Check sheet for the modelled part. Datum: model origin and axes. Units: mm. Face numbers are marked on the shaded views. Coordinates: 2 decimals unless noted, no trailing zeros. Order: outer loops, then holes, each group sorted by start corner. A loop starts at its lowest first (then second) coordinate and runs counter-clockwise, first axis right, second up.
1. Cross-section at A-A (z = 0). Count the separate pieces of the cut face and the enclosed holes in it, then the cut area to 3 significant figures.
2. Thickness scan on line 1 (Z direction, x = -1, y = -2.75); line 2 (Y direction, x = 33, z = 2); line 3 (Z direction, x = 76.2, y = 5). Record the ranges inside material, lowest first.
3. Cross-section at B-B (x = 76.2). Enter the section's corners in (y, z).
4. Draft check along Z on the marked faces 1 and 2. Enter one of: released by +Z, released by -Z, zero draft, split by the parting line, or undercut.
5. Cross-section at D-D (z = 7.5). Enter the section's corners in (x, y), then the cut area to 3 significant figures.
6. Gauge pin test, flat ends, axial feed: pin 1 Ø7.5 at (x, z) = (25.4, 0) entering from -Y; pin 2 Ø6.5 at (x, z) = (76.2, 23.81) entering from +Y; pin 3 Ø21 at (x, z) = (-3, 0.5) entering from +Y; pin 4 Ø2 at (x, z) = (-47, 25) entering from -Y. Record the tip position at first contact, or that the pin passes through.
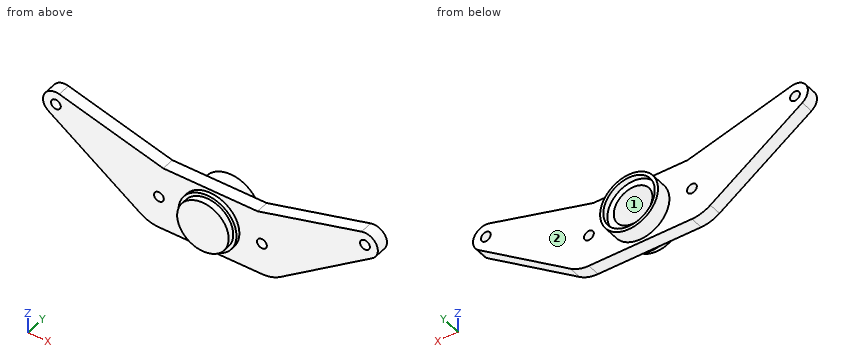
```python
from build123d import *

# Parameters (mm, degrees)
BOSS_EXTRUDE1_DEPTH    = 6.35
BOSS_EXTRUDE2_START    = -14.224
SKETCH2_R              = 14.2875
BOSS_EXTRUDE2_DEPTH    = 19.431
HOLE1_D                = 19.05
HOLE1_DEPTH            = 19.05
HOLE1_CBORE_D          = 25.4
HOLE1_CBORE_DEPTH      = 2.794
F_10_32_TAPPED_HOLE1_D = 4.826
SKETCH7_R              = 14.2875
SKETCH7_R_2            = 12.7
CUT_EXTRUDE1_DEPTH     = 3.175


with BuildPart() as part:
    # Sketch1 → Boss-Extrude1 (new body)
    with BuildSketch(Plane(origin=(0, 0, 0), x_dir=(1, 0, 0), z_dir=(0, 1, 0))):
        with BuildLine():
            Line((79.832170731, -18.603869107), (34.480426828, 13.021577233))
            ThreePointArc((34.480426828, 13.021577233), (30.159101093, 15.14485331), (25.4, 15.875))
            Line((25.4, 15.875), (-25.4, 15.875))
            ThreePointArc((-25.4, 15.875), (-30.159101093, 15.14485331), (-34.480426828, 13.021577233))
            Line((-34.480426828, 13.021577233), (-79.832170731, -18.603869107))
            ThreePointArc((-79.832170731, -18.603869107), (-81.949664243, -26.507655114), (-74.520111094, -29.936262999))
            Line((-74.520111094, -29.936262999), (-23.262053626, -15.875))
            Line((-23.262053626, -15.875), (23.262053626, -15.875))
            Line((23.262053626, -15.875), (74.520111094, -29.936262999))
            ThreePointArc((74.520111094, -29.936262999), (81.949664243, -26.507655114), (79.832170731, -18.603869107))
        make_face()
    extrude(amount=BOSS_EXTRUDE1_DEPTH)

    # Sketch2 → Boss-Extrude2 (add)
    with BuildSketch(Plane.XZ.offset(BOSS_EXTRUDE2_START)):
        Circle(SKETCH2_R)
    extrude(amount=BOSS_EXTRUDE2_DEPTH)

    # Hole1
    with Locations(Plane(origin=(0, 14.224, 0), x_dir=(1, 0, 0), z_dir=(0, 1, 0))):
        with Locations((0, 0)):
            CounterBoreHole(HOLE1_D / 2, HOLE1_CBORE_D / 2, HOLE1_CBORE_DEPTH, depth=HOLE1_DEPTH)

    # #10-32 Tapped Hole1 (through all)
    with Locations(Plane(origin=(0, 6.35, 0), x_dir=(1, 0, 0), z_dir=(0, 1, 0))):
        with Locations((-25.4, 0), (25.4, 0), (-76.2, -23.8125), (76.2, -23.8125)):
            Hole(F_10_32_TAPPED_HOLE1_D / 2)

    # Sketch7 → Cut-Extrude1 (cut)
    with BuildSketch(Plane.XZ.offset(5.207)):
        Circle(SKETCH7_R)
        Circle(SKETCH7_R_2, mode=Mode.SUBTRACT)
    extrude(amount=-CUT_EXTRUDE1_DEPTH, mode=Mode.SUBTRACT)


solid = part.part
```
Data:
1. separate pieces: 3
1. enclosed holes: 0
1. area: 597 mm2
2. line 1: z = -12.66 to -9.47, 9.47 to 12.66
2. line 2: y = 0 to 6.35
2. line 3: z = 16.07 to 21.4, 26.23 to 30.16
3. outline: (0, 16.07) - (6.35, 16.07) - (6.35, 21.4) - (0, 21.4) - close; (0, 26.23) - (6.35, 26.23) - (6.35, 30.16) - (0, 30.16) - close
4. face 1: undercut
4. face 2: zero draft
5. outline: (-63.91, 0) - (-12.16, 0) - (-12.16, -2.03) - (-10.25, -2.03) - (-10.25, -5.21) - (10.25, -5.21) - (10.25, -2.03) - (12.16, -2.03) - (12.16, 0) - (63.91, 0) - (63.91, 6.35) - (12.16, 6.35) - (12.16, 14.22) - (10.25, 14.22) - (10.25, 11.43) - (5.87, 11.43) - (5.87, -4.83) - (-5.87, -4.83) - (-5.87, 11.43) - (-10.25, 11.43) - (-10.25, 14.22) - (-12.16, 14.22) - (-12.16, 6.35) - (-63.91, 6.35) - close
5. area: 869 mm2
6. pin 1: stops at y = 0
6. pin 2: stops at y = 6.35
6. pin 3: stops at y = 14.22
6. pin 4: passes through
